For this review, take the finished solid that the model builds, in its own axes (mm). A direction names the side the tool comes from. Give positions to 0.01 mm unless a question says otherwise; leave off trailing zeros. Order: outer loops, then holes, each group sorted by start corner. A loop starts at its lowest first (then second) coordinate and runs counter-clockwise, first axis right, second up. Notation, with made-up numbers: (20, 74.5) - (44, 74.5) arc R23 cw to (44, 98.5) - close; hole circle Ø4 at (20, 6). An arc over 180 degrees is marked (long way). Put each result on its own line as item: value. Start each with the question number.
Autodesk Fusion 360 part; units mm, degrees
sketch "Sketch1" plane through (0, 0, 0) normal (0, 0, 1) x (1, 0, 0)
  line L0 (-30, 20) -> (-13, 20)
  line L1 (-13, 20) -> (-13, 7.5)
  line L2 (-13, 7.5) -> (-30, 7.5)
  line L3 (-30, 7.5) -> (-30, 20)
  dimension "d1" = 17
  dimension "d2" = 12.5
extrude "Extrude1" add sketch "Sketch1" along normal blind 6
fillet "Fillet1" radius 2 4 edges at (-21.5, 20, 6) (-13, 13.75, 6) (-30, 13.75, 6) (-21.5, 7.5, 6)
sketch "Sketch3" plane through (0, 0, 0) normal (0, 0, -1) x (-1, 0, 0)
  line L0 (13, 7.5) -> (30, 7.5)
  line L1 (30, 7.5) -> (30, 20)
  line L2 (30, 20) -> (13, 20)
  line L3 (13, 20) -> (13, 7.5)
  line L4 (13, 20) -> (30, 20)
  line L5 (30, 20) -> (30, 7.5)
  line L6 (30, 7.5) -> (13, 7.5)
  line L7 (13, 7.5) -> (13, 20)
  line L8 (12, 20) -> (31, 20)
  line L9 (12, 7.5) -> (31, 7.5)
  line L10 (12, 20) -> (31, 20)
  line L11 (31, 20) -> (31, 7.5)
  line L12 (31, 7.5) -> (12, 7.5)
  line L13 (12, 7.5) -> (12, 20)
  point P0 (21.5, 20)
  point P1 (21.5, 7.5)
  dimension "d10" = 19
  dimension "d11" = 19
extrude "Extrude3" add sketch "Sketch3" against normal blind 1 contours L3 L7 L8 L9 L10 L12 L13 | L1 L5 L8 L9 L10 L11 L12
1. Add section C-C, the plane z = 1.45. Give the boundary of the cut face in (x, y).
2. Add section A-A, the plane x = -27.5. Give the boundary of the cut face in (y, z), then the cut area to 3 significant figures.
3. Tool access review of faces 1 (the face through (-30.5, 13.8, 1)), 2 (the face through (-12, 13.7, 0.5)), 3 (the face through (-12.5, 13.8, 1)): name each direction out of +Z, -Z, +X, -X, +Y, -Y from which nothing blocks a thin tool from reaching the whole face with its end or side.
4. Wall thickness on line 1 (X direction, y = 14.5, z = 3.6); line 2 (Y direction, x = -27, z = 5.2); line 3 (Z direction, x = -29, y = 19.75): over which ranges is each line inside the solid? List them lowest first. Write a range as from..to.
5. Add section B-B, the plane y = 13.5. Give the boundary of the cut face in (x, z), then the cut area to 3 significant figures.
6. Add section D-D, the plane y = 18.75. Give the boundary of the cut face in (x, z).
7. Clearance check with flat-ended pins moving along their axes: pin 1 (0.5 mm diameter, centred on x = -30.5, y = 12.5, fed in from +Z); pin 2 (2.5 mm diameter, centred on y = 14.5, z = 3, fed in from +X). State where each tip first meets the part, or that it passes through.
Found:
1. outline: (-30, 7.5) - (-13, 7.5) - (-13, 20) - (-30, 20) - close
2. outline: (7.5, 0) - (20, 0) - (20, 4) arc R2 ccw to (18, 6) - (9.5, 6) arc R2 ccw to (7.5, 4) - close
2. area: 73.3 mm^2
3. face 1: +Z, -X, +Y, -Y
3. face 2: +Z, -Z, +X, +Y, -Y
3. face 3: +Z, +X, +Y, -Y
4. line 1: x = -30..-13
4. line 2: y = 7.9..19.6
4. line 3: z = 0..4.97
5. outline: (-31, 0) - (-12, 0) - (-12, 1) - (-13, 1) - (-13, 4) arc R2 ccw to (-15, 6) - (-28, 6) arc R2 ccw to (-30, 4) - (-30, 1) - (-31, 1) - close
5. area: 102 mm^2
6. outline: (-31, 0) - (-12, 0) - (-12, 1) - (-13, 1) - (-13, 4) arc R2 ccw to (-14.25, 5.85) - (-28.75, 5.85) arc R2 ccw to (-30, 4) - (-30, 1) - (-31, 1) - close
7. pin 1: stops at z = 1
7. pin 2: stops at x = -13
